```python
from build123d import *

# Parameters (mm, degrees)
F0_R     = 5
F1_DEPTH = 5
F2_DEPTH = 20
F3_R     = 5
F4_DEPTH = 25


with BuildPart() as f1:
    # F0 (on Top) → F1 (new body)
    with BuildSketch(Plane.XY):
        Polygon((-31.1052, 21.068258), (-31.1052, 0), (-18.978415, 0), (-18.978415, -7.215436), (-5.24761, -7.215436), (-5.24761, 21.068258), align=None)
        with Locations((-18.008273, 10.610935)):
            Circle(F0_R, mode=Mode.SUBTRACT)
    extrude(amount=F1_DEPTH)

    # F0 (on Top) → F2 (join)
    with BuildSketch(Plane.XY):
        Polygon((13.400096, 21.068258), (-5.24761, 21.068258), (-5.24761, -7.215436), (0, -7.215436), (0, 14.73404), (13.400096, 14.73404), align=None)
    extrude(amount=F2_DEPTH)

    # F3 (on Right) → F4 (cut)
    with BuildSketch(Plane.YZ):
        with Locations((3.955835, 13.019141)):
            Circle(F3_R)
    extrude(amount=-F4_DEPTH, mode=Mode.SUBTRACT)


solid = f1.part
```
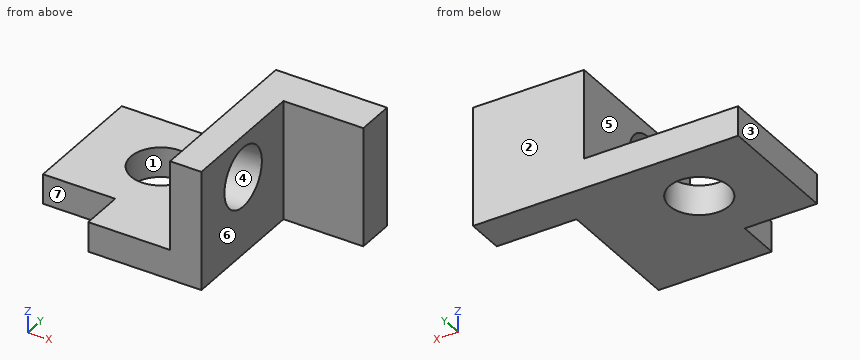
The model under review builds one solid part; all positions refer to its coordinate system, in mm. Face numbers are marked on the shaded views. A direction names the side the tool comes from. Give positions to 0.01 mm unless a question says otherwise; leave off trailing zeros. Write each loop counter-clockwise with the first axis right and the second up, starting at its lowest first coordinate (ties: lowest second). Pieces come first, ordered by that corner, then holes. Notation, with made-up numbers: M 24,-34 L 63,-34 A22 ccw 63,-24 Z; hole C -31.5,-0.5 d9. An arc over 180 degrees is marked long. Write item = value, one per line. Start each with the question number.
Q1. Machinability: for the marked faces 5, 6 and 7, which of the approach directions +Z, -Z, +X, -X, +Y, -Y give a long, thin tool a straight path to every point of the face, cutting with its end or side? Answer none if there is none.
Q2. For line 1 (Z direction, x = -9.5, y = 18.25); line 2 (Y direction, x = 2, z = 4.25); line 3 (X direction, y = 18.75, z = 5.75), list the stretches that pass through material, from the lowest coordinate up.
Q3. Clearance check with flat-ended pins moving along their axes: pin 1 (10 mm diameter, centred on y = 1, z = 11.5, fed in from +X); pin 2 (13 mm diameter, centred on x = -18.01, y = 10.61, fed in from +Z); pin 3 (5.5 mm diameter, centred on y = -4, z = 3.5, fed in from -X); pin 4 (5 mm diameter, centred on x = -21, z = 8.5, fed in from -Y). State where each tip first meets the part, or that it passes through.
Q4. We need section B-B (x = -19.5). State the section outline as (y, z) points, plus the area to 3 significant figures.
Q5. Mouldability with a two-part tool opening along Y and no side actions: class the marked faces 1, 2, 3 and 4 as released by +Y, released by -Y, zero draft, split by the parting line, or undercut.
Q6. We need section C-C (y = 12.25). State the section outline as (x, z) points.
Q7. We need section D-D (z = 2.5). State the section outline as (x, y) points, plus the area to 3 significant figures.
Q8. We need section A-A (z = 11). State the section outline as (x, y) points.
Result set:
q1.face_5 = +Z, -X, +Y, -Y
q1.face_6 = +Z, -Z, +X, -Y
q1.face_7 = +Z, -Z, -X, -Y
q2.line_1 = 0 to 5
q2.line_2 = 14.73 to 21.07
q2.line_3 = -5.25 to 13.4
q3.pin_1 = 0
q3.pin_2 = 5
q3.pin_3 = -18.98
q3.pin_4 = through
q4.outline = M 0,0 L 5.84,0 L 5.84,5 L 0,5 Z; M 15.38,0 L 21.07,0 L 21.07,5 L 15.38,5 Z
q4.area = 57.6 mm2
q5.face_1 = undercut
q5.face_2 = released by +Y
q5.face_3 = zero draft
q5.face_4 = undercut
q6.outline = M -31.11,0 L -22.73,0 L -22.73,5 L -31.11,5 Z; M -13.28,0 L 0,0 L 0,20 L -5.25,20 L -5.25,5 L -13.28,5 Z
q7.outline = M -31.11,0 L -18.98,0 L -18.98,-7.22 L 0,-7.22 L 0,14.73 L 13.4,14.73 L 13.4,21.07 L -31.11,21.07 Z; hole C -18.01,10.61 d10
q7.area = 799 mm2
q8.outline = M -5.25,-7.22 L 0,-7.22 L 0,-0.62 L -5.25,-0.62 Z; M -5.25,8.53 L 0,8.53 L 0,14.73 L 13.4,14.73 L 13.4,21.07 L -5.25,21.07 Z
